```python
from build123d import *

# Parameters (mm, degrees)
SKETCH_1_R      = 34
SKETCH_1_R_2    = 16.55
EXTRUDE_1_DEPTH = 2.5


with BuildPart() as part:
    # 草图1 → 凸台-拉伸1 (new body)
    with BuildSketch(Plane(origin=(0, 2.5, 0), x_dir=(1, 0, 0), z_dir=(0, 1, 0))):
        Circle(SKETCH_1_R)
        Circle(SKETCH_1_R_2, mode=Mode.SUBTRACT)
        with BuildLine():
            Line((-3, -22.449944321), (-3, -27.549954628))
            ThreePointArc((-3, -27.549954628), (-3.718260111, -29.085253575), (-5.357142857, -29.51780853))
            ThreePointArc((-5.357142857, -29.51780853), (-21.213203436, -21.213203436), (-29.51780853, -5.357142857))
            ThreePointArc((-29.51780853, -5.357142857), (-29.085253575, -3.718260111), (-27.549954628, -3))
            Line((-27.549954628, -3), (-22.449944321, -3))
            ThreePointArc((-22.449944321, -3), (-21.198857836, -3.439621005), (-20.497775249, -4.565217391))
            ThreePointArc((-20.497775249, -4.565217391), (-14.849242405, -14.849242405), (-4.565217391, -20.497775249))
            ThreePointArc((-4.565217391, -20.497775249), (-3.439621005, -21.198857836), (-3, -22.449944321))
        make_face(mode=Mode.SUBTRACT)
        with BuildLine():
            Line((-22.449944321, 3), (-27.549954628, 3))
            ThreePointArc((-27.549954628, 3), (-29.085253575, 3.718260111), (-29.51780853, 5.357142857))
            ThreePointArc((-29.51780853, 5.357142857), (-21.213203436, 21.213203436), (-5.357142857, 29.51780853))
            ThreePointArc((-5.357142857, 29.51780853), (-3.718260111, 29.085253575), (-3, 27.549954628))
            Line((-3, 27.549954628), (-3, 22.449944321))
            ThreePointArc((-3, 22.449944321), (-3.439621005, 21.198857836), (-4.565217391, 20.497775249))
            ThreePointArc((-4.565217391, 20.497775249), (-14.849242405, 14.849242405), (-20.497775249, 4.565217391))
            ThreePointArc((-20.497775249, 4.565217391), (-21.198857836, 3.439621005), (-22.449944321, 3))
        make_face(mode=Mode.SUBTRACT)
        with BuildLine():
            Line((3, 22.449944321), (3, 27.549954628))
            ThreePointArc((3, 27.549954628), (3.718260111, 29.085253575), (5.357142857, 29.51780853))
            ThreePointArc((5.357142857, 29.51780853), (21.213203436, 21.213203436), (29.51780853, 5.357142857))
            ThreePointArc((29.51780853, 5.357142857), (29.085253575, 3.718260111), (27.549954628, 3))
            Line((27.549954628, 3), (22.449944321, 3))
            ThreePointArc((22.449944321, 3), (21.198857836, 3.439621005), (20.497775249, 4.565217391))
            ThreePointArc((20.497775249, 4.565217391), (14.849242405, 14.849242405), (4.565217391, 20.497775249))
            ThreePointArc((4.565217391, 20.497775249), (3.439621005, 21.198857836), (3, 22.449944321))
        make_face(mode=Mode.SUBTRACT)
        with BuildLine():
            Line((22.449944321, -3), (27.549954628, -3))
            ThreePointArc((27.549954628, -3), (29.085253575, -3.718260111), (29.51780853, -5.357142857))
            ThreePointArc((29.51780853, -5.357142857), (21.213203436, -21.213203436), (5.357142857, -29.51780853))
            ThreePointArc((5.357142857, -29.51780853), (3.718260111, -29.085253575), (3, -27.549954628))
            Line((3, -27.549954628), (3, -22.449944321))
            ThreePointArc((3, -22.449944321), (3.439621005, -21.198857836), (4.565217391, -20.497775249))
            ThreePointArc((4.565217391, -20.497775249), (14.849242405, -14.849242405), (20.497775249, -4.565217391))
            ThreePointArc((20.497775249, -4.565217391), (21.198857836, -3.439621005), (22.449944321, -3))
        make_face(mode=Mode.SUBTRACT)
    extrude(amount=-EXTRUDE_1_DEPTH)


solid = part.part
```
Design review of the part built by this model. Coordinates are the model's own, in mm. Round coordinates to 2 decimals unless told otherwise and drop trailing zeros. Write each loop counter-clockwise with the first axis right and the second up, starting at its lowest first coordinate (ties: lowest second). Pieces come first, ordered by that corner, then holes. Notation, with made-up numbers: (38.25, 71.5) -> (91.25, 71.5) arc R22 cw to (91.25, 93.5) -> close; hole circle Ø8 at (-16.75, 30). An arc over 180 degrees is marked (long way). Answer in a Markdown table with one row per item.
Q1. Draft analysis for pull direction X (two halves, no side actions). For faces 1 (the face through (-3.452, 1.268, 21.184)), 2 (the face through (15, 0, -8)), 3 (the face through (18.28, 1.27, -28.67)), state which applies: +X half, -X half, draft (parallel to the pull), parting line (faces both ways), or undercut.
The answers:
| item | result |
|---|---|
| face 1 | undercut |
| face 2 | draft |
| face 3 | parting line |
Q2. Take a section at B-B, the plane z = 0. State the section outline as (x, y) points, then the cut area to 4 significant figures.
The answers:
| item | result |
|---|---|
| outline | (-34, 0) -> (-16.55, 0) -> (-16.55, 2.5) -> (-34, 2.5) -> close; (16.55, 0) -> (34, 0) -> (34, 2.5) -> (16.55, 2.5) -> close |
| area | 87.25 mm² |
Q3. Clearance check with flat-ended pins moving along their axes: pin 1 Ø1.5 at (y, z) = (1, -1.5) entering from -X; pin 2 Ø1 at (y, z) = (0.5, 24) entering from +X; pin 3 Ø0.8 at (y, z) = (1.5, -25) entering from +X. State where each tip first meets the part, or that it passes through.
The answers:
| item | result |
|---|---|
| pin 1 | x = -33.99 |
| pin 2 | x = 24.57 |
| pin 3 | x = 23.47 |
Q4. Take a section at D-D, the plane z = 14. State the section outline as (x, y) points, then the cut area to 3 significant figures.
The answers:
| item | result |
|---|---|
| outline | (-30.98, 0) -> (-26.53, 0) -> (-26.53, 2.5) -> (-30.98, 2.5) -> close; (-15.65, 0) -> (-8.83, 0) -> (-8.83, 2.5) -> (-15.65, 2.5) -> close; (8.83, 0) -> (15.65, 0) -> (15.65, 2.5) -> (8.83, 2.5) -> close; (26.53, 0) -> (30.98, 0) -> (30.98, 2.5) -> (26.53, 2.5) -> close |
| area | 56.4 mm² |
Q5. To check wall thickness, follow L1, parallel to Z at x = 0, y = 1.7; L2, parallel to X at y = 1.2, z = 12; L3, parallel to Z at x = 19, y = 0.25. State the ranges of each line that lie inside material, in increasing order. Write a range as [from, to].
The answers:
| item | result |
|---|---|
| L1 | [-34, -16.55], [16.55, 34] |
| L2 | [-31.81, -27.5], [-17.23, -11.4], [11.4, 17.23], [27.5, 31.81] |
| L3 | [-28.2, -23.22], [-8.94, 8.94], [23.22, 28.2] |
Q6. Take a section at A-A, the plane x = 0. State the section outline as (y, z) points, then the cut area to 4 significant figures.
The answers:
| item | result |
|---|---|
| outline | (0, -34) -> (2.5, -34) -> (2.5, -16.55) -> (0, -16.55) -> close; (0, 16.55) -> (2.5, 16.55) -> (2.5, 34) -> (0, 34) -> close |
| area | 87.25 mm² |
Q7. Take a section at C-C, the plane y = 0.4. Count the separate pieces of the cut face and the enclosed holes in it, then the cut area to 3 significant figures.
The answers:
| item | result |
|---|---|
| separate pieces | 1 |
| enclosed holes | 5 |
| area | 1,560 mm² |
